from build123d import *

# Parameters (mm, degrees)
BOX006_W          = 3
BOX006_H          = 120
BOX006_DEPTH      = 4
BOX005_W          = 10
BOX005_H          = 128
BOX005_DEPTH      = 4
BOX004_W          = 4
BOX004_H          = 40
BOX004_DEPTH      = 100
CYLINDER010_R     = 6.2
CYLINDER010_DEPTH = 3
CYLINDER009_R     = 6.2
CYLINDER009_DEPTH = 3
CYLINDER001_R     = 3.2
CYLINDER001_DEPTH = 6.5
CYLINDER_R        = 3.2
CYLINDER_DEPTH    = 6.5
BOX_W             = 22
BOX_H             = 80
BOX_DEPTH         = 6.5
BOX002_W          = 8
BOX002_H          = 4
BOX002_DEPTH      = 1
BOX001_W          = 8
BOX001_H          = 4
BOX001_DEPTH      = 1
BOX003_W          = 8
BOX003_H          = 52
BOX003_DEPTH      = 1
CHAMFER_SIZE      = 3
CHAMFER001_SIZE   = 1
CHAMFER002_SIZE   = 1
CHAMFER003_SIZE   = 0.6


with BuildPart() as cube006:
    # Box006 → Box006 (new body)
    with BuildSketch(Plane(origin=(17, -20, 96), x_dir=(1, 0, 0), z_dir=(0, 0, 1))):
        with Locations((1.5, 60)):
            Rectangle(BOX006_W, BOX006_H)
    extrude(amount=BOX006_DEPTH)


with BuildPart() as cube005:
    # Box005 → Box005 (new body)
    with BuildSketch(Plane(origin=(14, -24, 96), x_dir=(1, 0, 0), z_dir=(0, 0, 1))):
        with Locations((5, 64)):
            Rectangle(BOX005_W, BOX005_H)
    extrude(amount=BOX005_DEPTH)


with BuildPart() as cut005:
    # Box004 → Box004 (new body)
    with BuildSketch(Plane(origin=(20, 20, 0), x_dir=(1, 0, 0), z_dir=(0, 0, 1))):
        with Locations((2, 20)):
            Rectangle(BOX004_W, BOX004_H)
    extrude(amount=BOX004_DEPTH)

    # Fusion012: union Cube005
    add(cube005.part)

    # Cut005: cut Cube006
    add(cube006.part, mode=Mode.SUBTRACT)


with BuildPart() as cylinder010:
    # Cylinder010 → Cylinder010 (new body)
    with BuildSketch(Plane(origin=(10, 71, 3.5), x_dir=(1, 0, 0), z_dir=(0, 0, 1))):
        Circle(CYLINDER010_R)
    extrude(amount=CYLINDER010_DEPTH)


with BuildPart() as cylinder009:
    # Cylinder009 → Cylinder009 (new body)
    with BuildSketch(Plane(origin=(10, 9, 3.5), x_dir=(1, 0, 0), z_dir=(0, 0, 1))):
        Circle(CYLINDER009_R)
    extrude(amount=CYLINDER009_DEPTH)


with BuildPart() as cylinder001:
    # Cylinder001 → Cylinder001 (new body)
    with BuildSketch(Plane(origin=(10, 71, -3), x_dir=(1, 0, 0), z_dir=(0, 0, 1))):
        Circle(CYLINDER001_R)
    extrude(amount=CYLINDER001_DEPTH)


with BuildPart() as cylinder:
    # Cylinder → Cylinder (new body)
    with BuildSketch(Plane(origin=(10, 9, -3), x_dir=(1, 0, 0), z_dir=(0, 0, 1))):
        Circle(CYLINDER_R)
    extrude(amount=CYLINDER_DEPTH)


with BuildPart() as cut004:
    # Box → Box (new body)
    with BuildSketch(Plane(origin=(2, 0, 0), x_dir=(1, 0, 0), z_dir=(0, 0, 1))):
        with Locations((11, 40)):
            Rectangle(BOX_W, BOX_H)
    extrude(amount=BOX_DEPTH)

    # Cut: cut Cylinder
    add(cylinder.part, mode=Mode.SUBTRACT)

    # Cut002: cut Cylinder001
    add(cylinder001.part, mode=Mode.SUBTRACT)

    # Cut003: cut Cylinder009
    add(cylinder009.part, mode=Mode.SUBTRACT)

    # Cut004: cut Cylinder010
    add(cylinder010.part, mode=Mode.SUBTRACT)


with BuildPart() as cube002:
    # Box002 → Box002 (new body)
    with BuildSketch(Plane(origin=(6, 76, -1), x_dir=(1, 0, 0), z_dir=(0, 0, 1))):
        with Locations((4, 2)):
            Rectangle(BOX002_W, BOX002_H)
    extrude(amount=BOX002_DEPTH)


with BuildPart() as fusion010:
    # Box001 → Box001 (new body)
    with BuildSketch(Plane(origin=(6, 0, -1), x_dir=(1, 0, 0), z_dir=(0, 0, 1))):
        with Locations((4, 2)):
            Rectangle(BOX001_W, BOX001_H)
    extrude(amount=BOX001_DEPTH)

    # Fusion010: union Cube002
    add(cube002.part)


with BuildPart() as chamfer003:
    # Box003 → Box003 (new body)
    with BuildSketch(Plane(origin=(6, 14, -1), x_dir=(1, 0, 0), z_dir=(0, 0, 1))):
        with Locations((4, 26)):
            Rectangle(BOX003_W, BOX003_H)
    extrude(amount=BOX003_DEPTH)

    # Fusion011: union Fusion010
    add(fusion010.part)

    # Fusion: union Cut004
    add(cut004.part)

    # Fusion013: union Cut005
    add(cut005.part)

    # Chamfer
    chamfer_edges = [chamfer003.edges().sort_by_distance(p)[0] for p in [
        (2, 0, 3.25),
        (2, 80, 3.25),
        (24, 0, 3.25),
        (24, 80, 3.25),
        (24, 104, 98),
        (24, -24, 98),
        (14, -24, 98),
        (14, 104, 98),
    ]]
    chamfer(chamfer_edges, length=CHAMFER_SIZE)

    # Chamfer001
    chamfer001_edges = [chamfer003.edges().sort_by_distance(p)[0] for p in [
        (20, 0, 96),
        (18.5, -20, 96),
        (17, 40, 96),
        (18.5, 100, 96),
        (20, 80, 96),
        (20, 80, 100),
        (20, 40, 100),
        (20, 0, 100),
        (18.5, 100, 100),
        (17, 40, 100),
        (18.5, -20, 100),
    ]]
    chamfer(chamfer001_edges, length=CHAMFER001_SIZE)

    # Chamfer002
    chamfer002_edges = [chamfer003.edges().sort_by_distance(p)[0] for p in [
        (13, 80, 6.5),
        (3.5, 78.5, 6.5),
        (2, 40, 6.5),
        (3.5, 1.5, 6.5),
        (13, 0, 6.5),
        (22.5, 1.5, 6.5),
        (24, 11.5, 6.5),
        (24, 68.5, 6.5),
        (22.5, 78.5, 6.5),
    ]]
    chamfer(chamfer002_edges, length=CHAMFER002_SIZE)

    # Chamfer003
    chamfer003_edges = [chamfer003.edges().sort_by_distance(p)[0] for p in [
        (6, 2, -1),
        (10, 4, -1),
        (14, 2, -1),
        (14, 78, -1),
        (10, 76, -1),
        (6, 78, -1),
        (6, 40, -1),
        (10, 66, -1),
        (14, 40, -1),
        (10, 14, -1),
        (10, 0, -1),
        (10, 80, -1),
    ]]
    chamfer(chamfer003_edges, length=CHAMFER003_SIZE)


solid = chamfer003.part
Work out the finished part from the listing and answer in its coordinate system (mm). A direction names the side the tool comes from. Coordinates: 2 decimals unless noted, no trailing zeros. Order: outer loops, then holes, each group sorted by start corner. A loop starts at its lowest first (then second) coordinate and runs counter-clockwise, first axis right, second up. Notation, with made-up numbers: (-27.5, -32) - (26.5, -32) arc R15 ccw to (26.5, -8) - close; hole circle Ø4 at (-23, 71.5). An arc over 180 degrees is marked (long way). Put each result on its own line as item: value. Start each with the question number.
1) Find section C-C (x = 10). State how many separate pieces and enclosed holes the cut face has, plus the area to 3 significant figures.
2) For faces 1 (the flat face through (13, 0, 3)), 2 (the flat face through (13, 80, 3)), 3 (the cylindrical face through (8.656, 2.947, 4.979)), 4 (the flat face through (10, 2, -1)), 5 (the flat face through (14, 39, 98)), determine the directions among +Z, -Z, +X, -X, +Y, -Y from which every point of the face is accessible in a straight line to the end or side of a thin tool.
3) Find the intervals of material crossed by line 1 (Y direction, x = 10, z = 4.2); line 2 (X direction, y = 9, z = 2.1); line 3 (Z direction, x = 18.5, y = 63.5), in increasing order. Write a range as from..to.
4) Flat-ended cylindrical pins translate along their axes: pin 1 (3 mm diameter, centred on x = 21.5, z = 49.5, fed in from -Y); pin 2 (7.5 mm diameter, centred on x = 10, y = 71, fed in from +Z); pin 3 (5 mm diameter, centred on x = 20.5, y = 33.5, fed in from -Z); pin 4 (10 mm diameter, centred on x = 10, y = 68.5, fed in from +Z). Find the tip coordinate at first contact, or state that the pin passes through.
5) Find section D-D (z = 8). Give the vertices of the cut face in (x, y), plus the area to 3 significant figures.
6) Find section B-B (y = 35.5). Give the vertices of the cut face in (x, z), plus the area to 3 significant figures.
7) Find section A-A (y = 9). Give the vertices of the cut face in (x, z), plus the area to 3 significant figures.
8) For a pull along X with two mould halves and no side action, classify faces 6 (the flat face through (19, -24, 98)), 7 (the flat face through (3, 78, 3)), 8 (the flat face through (13, 6, 3.5)) as released by +X, released by -X, zero draft, split by the parting line, or undercut.
Results list:
1. separate pieces: 3
1. enclosed holes: 0
1. area: 459 mm^2
2. face 1: -Z, +X, -X, -Y
2. face 2: -Z, +X, -X, +Y
2. face 3: none
2. face 4: -Z, +X, -X, +Y, -Y
2. face 5: +Z, -X, +Y, -Y
3. line 1: y = 0..2.8, 15.2..64.8, 77.2..80
3. line 2: x = 2..6.8, 13.2..24
3. line 3: z = 0..6.5
4. pin 1: stops at y = 20
4. pin 2: stops at z = 3.5
4. pin 3: stops at z = 0
4. pin 4: stops at z = 100
5. outline: (20, 20) - (24, 20) - (24, 60) - (20, 60) - close
5. area: 160 mm^2
6. outline: (2, 0) - (6, 0) - (6, -0.4) - (6.6, -1) - (13.4, -1) - (14, -0.4) - (14, 0) - (24, 0) - (24, 100) - (21, 100) - (20, 99) - (20, 6.5) - (3, 6.5) - (2, 5.5) - close; (14, 96) - (16, 96) - (17, 97) - (17, 99) - (16, 100) - (14, 100) - close
6. area: 535 mm^2
7. outline: (2, 0) - (6.8, 0) - (6.8, 3.5) - (3.8, 3.5) - (3.8, 6.5) - (3, 6.5) - (2, 5.5) - close; (13.2, 0) - (24, 0) - (24, 5.5) - (23, 6.5) - (16.2, 6.5) - (16.2, 3.5) - (13.2, 3.5) - close; (14, 96) - (16, 96) - (17, 97) - (17, 99) - (16, 100) - (14, 100) - close; (20, 97) - (21, 96) - (24, 96) - (24, 100) - (21, 100) - (20, 99) - close
7. area: 108 mm^2
8. face 6: zero draft
8. face 7: released by -X
8. face 8: undercut
